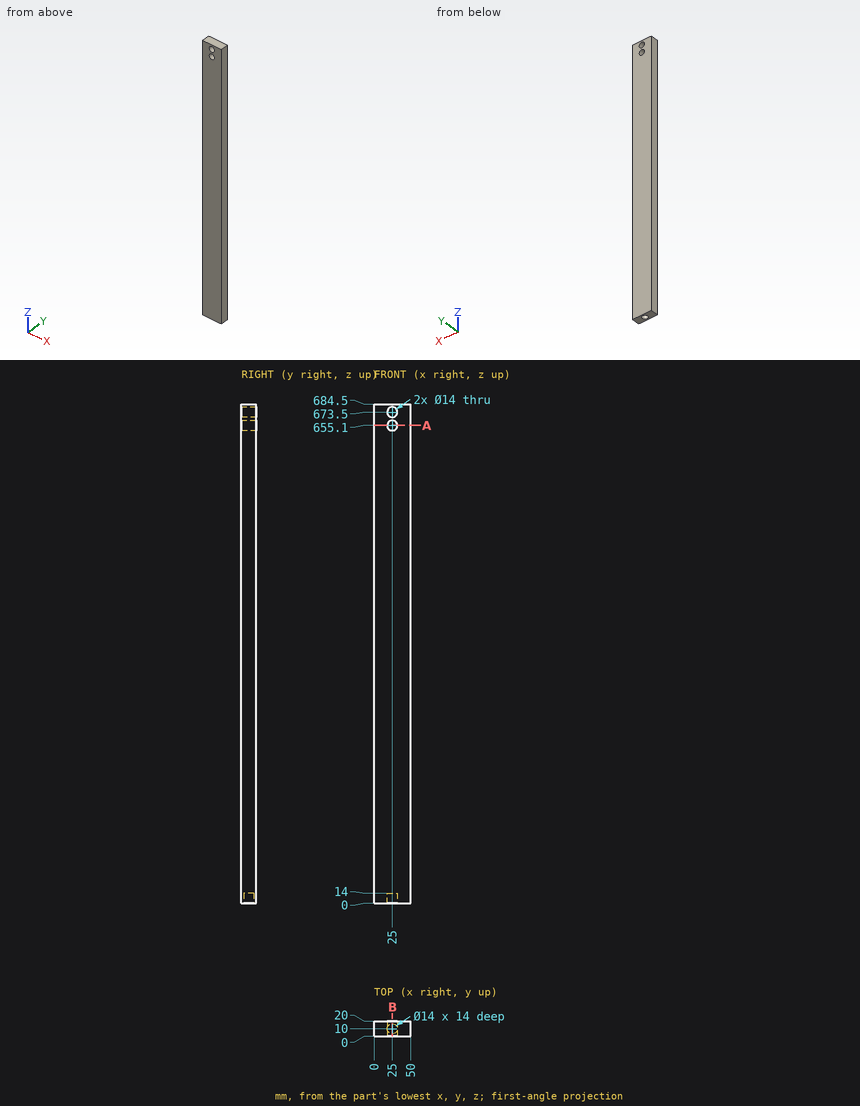
Input: dimensioned drawing with shaded views. Units: mm. Origin: part minimum x, y, z. Coordinates: 2 decimals unless noted, no trailing zeros. Loops run counter-clockwise (first coordinate to the right, second up) from the corner with the lowest first, then second, coordinate; pieces in that order, holes last. Notation, with made-up numbers: M 10,19.25 L 69,19.25 A19 cw 69,32.25 Z; hole C 23.25,68 d4. An arc over 180 degrees is marked long. Use a Markdown table: item, result. Add a question column.
Q1. Section query A-A, the plane z = 655.1. Return loops of the section in (x, y).
Q2. Material intervals for L1, parallel to Z at x = 25, y = 8.5; L2, parallel to Y at x = 25, z = 7; L3, parallel to Z at x = 19, y = 1.5, sorted ascending.
Q3. Section query B-B, the plane x = 25. Return loops of the section in (y, z).
Q4. First-contact query: pin 1 (4 mm diameter, centred on x = 32.5, y = 17.5, fed in from -Z). Flat tip, straight axial feed; report the tip coordinate or a pass-through.
Result:
| question | item | result |
|---|---|---|
| 1 | outline | M 0,0 L 18,0 L 18,20 L 0,20 Z; M 32,0 L 50,0 L 50,20 L 32,20 Z |
| 2 | L1 | z = 14 to 648.1, 662.1 to 666.5, 680.5 to 684.5 |
| 2 | L2 | y = 0 to 3, 17 to 20 |
| 2 | L3 | z = 0 to 651.49, 658.71 to 669.89, 677.11 to 684.5 |
| 3 | outline | M 0,0 L 3,0 L 3,14 L 17,14 L 17,0 L 20,0 L 20,648.1 L 0,648.1 Z; M 0,662.1 L 20,662.1 L 20,666.5 L 0,666.5 Z; M 0,680.5 L 20,680.5 L 20,684.5 L 0,684.5 Z |
| 4 | pin 1 | stops at z = 0 |
